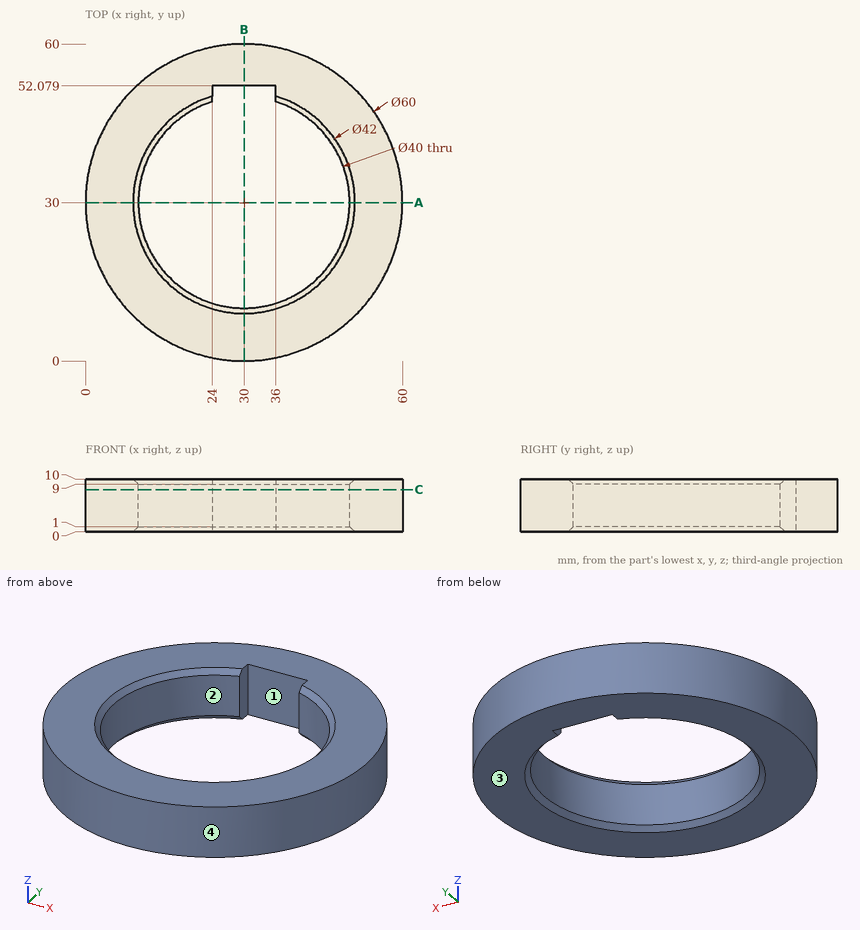
Geometry check sheet. Reference: drawing and pictorial views, mm from the part's lowest x, y, z. Round coordinates to 2 decimals unless told otherwise and drop trailing zeros. Write each loop counter-clockwise with the first axis right and the second up, starting at its lowest first coordinate (ties: lowest second). Pieces come first, ordered by that corner, then holes.
1. Section check B-B on x = 30. Enter the section's corners in (y, z).
2. Section check A-A on y = 30. Enter the section's corners in (x, z), plus the area to 3 significant figures.
3. Gauge pin test, flat ends, axial feed: P1, Ø0.9, axis at y = 50.5, z = 5, coming from the -X side; P2, Ø4, axis at x = 11.5, y = 27, coming from the +Z side; P3, Ø24, axis at x = 30, y = 30, coming from the -Z side; P4, Ø3, axis at x = 42, z = 6.5, coming from the -Y side. Record the tip position at first contact, or that the pin passes through.
4. Draft check along Y on the marked faces 1, 2, 3 and 4. Enter one of: +Y half, -Y half, draft (parallel to the pull), parting line (faces both ways), or undercut.
5. Section check C-C on z = 8. Enter the section's corners in (x, y).
6. Scan lines: L1, parallel to Y at x = 30, z = 6.5; L2, parallel to X at y = 30.5, z = 5.75; L3, parallel to Y at x = 18, z = 9.25 (1 decimal). Record each from-to range of solid material in increasing order.
Answer:
1. outline: (0, 0) - (9, 0) - (10, 1) - (10, 9) - (9, 10) - (0, 10) - close; (52.08, 0) - (60, 0) - (60, 10) - (52.08, 10) - close
2. outline: (0, 0) - (9, 0) - (10, 1) - (10, 9) - (9, 10) - (0, 10) - close; (50, 1) - (51, 0) - (60, 0) - (60, 10) - (51, 10) - (50, 9) - close
2. area: 198 mm2
3. P1: stops at x = 7.68
3. P2: stops at z = 9.74
3. P3: passes through
3. P4: stops at y = 1.9
4. face 1: undercut
4. face 2: undercut
4. face 3: draft
4. face 4: parting line
5. outline: circle Ø60 at (30, 30); hole (24, 49.08) arc R20 ccw (long way) to (36, 49.08) - (36, 52.08) - (24, 52.08) - close
6. L1: y = 0 to 10, 52.08 to 60
6. L2: x = 0 to 10.01, 49.99 to 60
6. L3: y = 2.5 to 13.7, 46.3 to 57.5
